Verification items for this drawing (mm, ordinates from the low corner). Give positions to 0.01 mm unless a question says otherwise; leave off trailing zeros. Loops run counter-clockwise (first coordinate to the right, second up) from the corner with the lowest first, then second, coordinate; pieces in that order, holes last. Notation, with made-up numbers: (71, -31.5) -> (89, -31.5) arc R12 ccw to (89, -12.5) -> close; hole circle Ø9 at (5, 34.5). An arc over 180 degrees is marked (long way). Answer as CSV lines item,"result". Start each with the question number.
(1) Section check A-A on y = 10.25. Enter the section's corners in (x, z) (3 decimals), plus the area to 3 significant figures.
(2) Gauge pin test, flat ends, axial feed: pin 1 Ø5 at (y, z) = (4.5, 101.5) entering from -X; pin 2 Ø5 at (y, z) = (8, 52) entering from +X; pin 3 Ø1 at (y, z) = (4, 72.5) entering from -X. Record the tip position at first contact, or that the pin passes through.
(3) Material ranges on line 1 (X direction, y = 13.25, z = 58.5); line 2 (Y direction, x = 14.5, z = 86) (3 decimals); line 3 (Z direction, x = 16.5, y = 4.5), recorded low to high. Write a range as from..to.
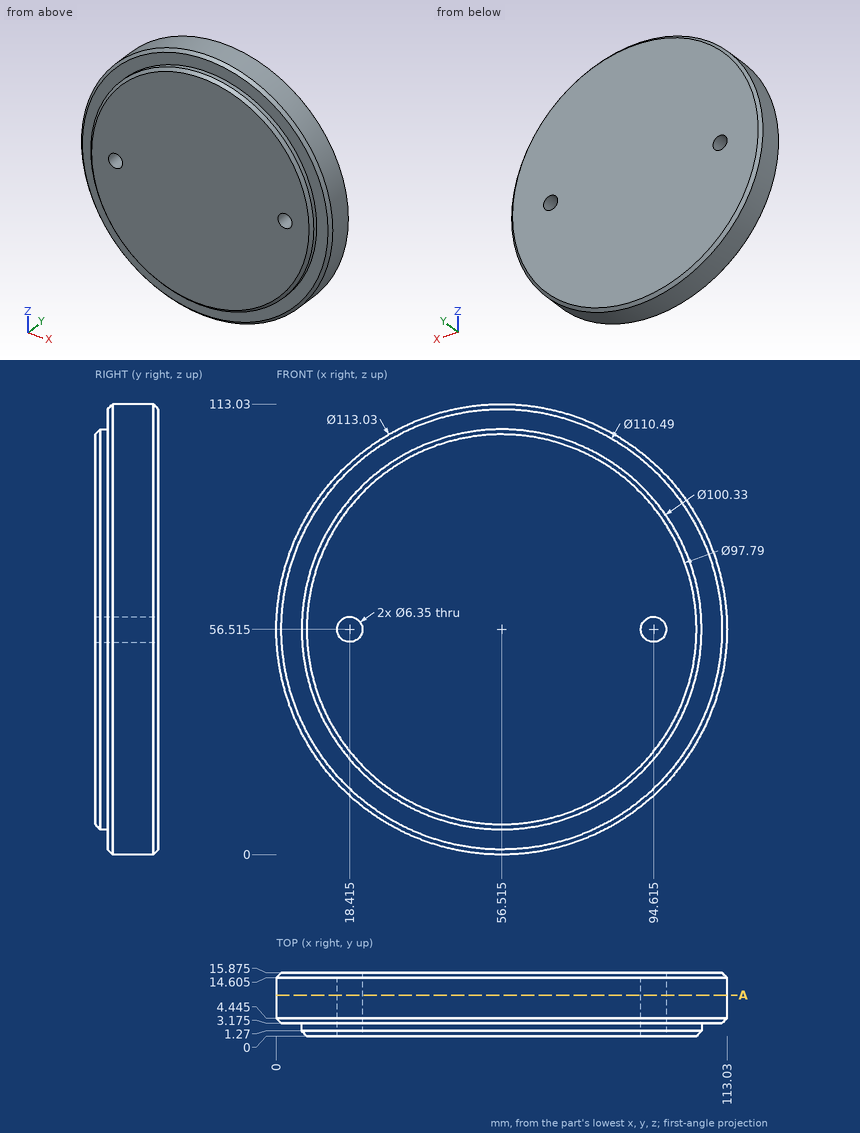
Working result:
1,outline,"circle Ø113.03 at (56.515, 56.515); hole circle Ø6.35 at (18.415, 56.515); hole circle Ø6.35 at (94.615, 56.515)"
1,area,"9,970 mm^2"
2,pin 1,"stops at x = 19.25"
2,pin 2,"stops at x = 112.99"
2,pin 3,"stops at x = 2.24"
3,line 1,"x = 0.03..15.94, 20.89..92.14, 97.09..113"
3,line 2,"y = 3.175..15.875"
3,line 3,"z = 16.61..53.98, 59.05..96.42"
